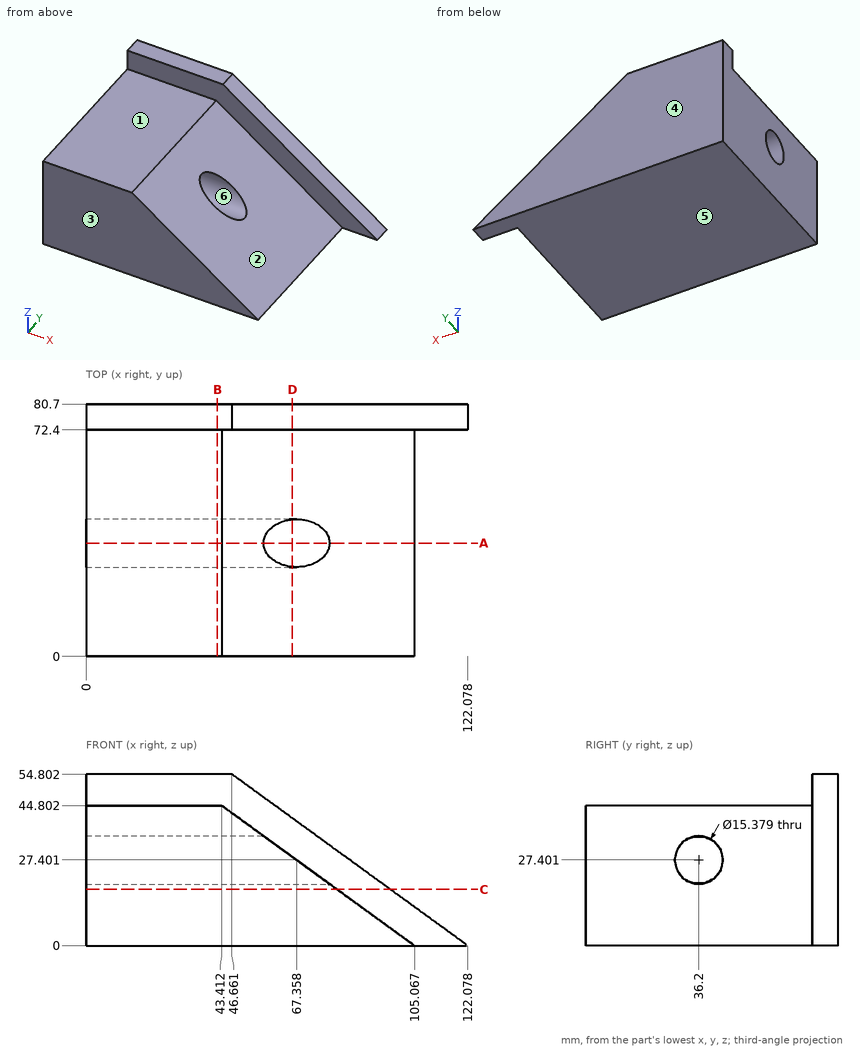
Input: dimensioned drawing with shaded views. Units: mm. Origin: part minimum x, y, z. A direction names the side the tool comes from. Round coordinates to 2 decimals unless told otherwise and drop trailing zeros. Order: outer loops, then holes, each group sorted by start corner. A loop starts at its lowest first (then second) coordinate and runs counter-clockwise, first axis right, second up. Notation, with made-up numbers: (6.25, 24.25) -> (15.25, 24.25) arc R16 cw to (15.25, 35.25) -> close; hole circle Ø7 at (-2, 69). An arc over 180 degrees is marked (long way). One line per item, written item: value. Start each with the question number.
Q1. Access query for the marked faces 1, 2 and 3. Directions: +Z, -Z, +X, -X, +Y, -Y. A direction counts if a zero-diameter tool reaches every point of the face in a straight line with its end or side. Return the directions, or none.
Q2. Section query D-D (x = 66). Return the cut outline in (y, z).
Q3. Draft query along Y for the marked faces 4, 5 and 6. Return one class per face: pulls with the +Y half, pulls with the -Y half, needs draft (parallel to the pull), parting line crosses it, or undercut.
Q4. Material intervals for probe 1 along Z at (x, y) = (42, 36.2); probe 2 along Z at (x, y) = (9, 66); probe 3 along Y at (x, z) = (55.5, 24) (1 decimal), sorted ascending.
Q5. Section query A-A (y = 36.2). Return the cut outline in (x, z), plus the area to 3 significant figures.
Q6. Section query B-B (x = 42). Return the cut outline in (y, z).
Q7. Pin query (flat end, axial travel): pin 1 (21.5 mm diameter, centred on x = 32, y = 45, fed in from +Z). Return the tip coordinate at first contact, or that it passes through.
Q8. Section query C-C (z = 18). Return the cut outline in (x, y) (1 decimal), plus the area to 3 significant figures.
Findings below:
1. face 1: +Z, +X, -X, -Y
1. face 2: +Z, +X, -Y
1. face 3: +Z, -Z, +X, -X, -Y
2. outline: (0, 0) -> (80.7, 0) -> (80.7, 40.75) -> (72.4, 40.75) -> (72.4, 28.39) -> (43.83, 28.39) arc R7.69 cw (long way) to (28.57, 28.39) -> (0, 28.39) -> close
3. face 4: pulls with the +Y half
3. face 5: needs draft
3. face 6: undercut
4. probe 1: 0 to 19.71, 35.09 to 44.8
4. probe 2: 0 to 44.8
4. probe 3: 0 to 29.3, 43.1 to 80.7
5. outline: (0, 0) -> (105.07, 0) -> (77.94, 19.71) -> (0, 19.71) -> close; (0, 35.09) -> (56.78, 35.09) -> (43.41, 44.8) -> (0, 44.8) -> close
5. area: 2,290 mm²
6. outline: (0, 0) -> (80.7, 0) -> (80.7, 54.8) -> (72.4, 54.8) -> (72.4, 44.8) -> (0, 44.8) -> close; hole circle Ø15.38 at (36.2, 27.4)
7. pin 1: z = 44.8
8. outline: (0, 0) -> (80.3, 0) -> (80.3, 72.4) -> (97.3, 72.4) -> (97.3, 80.7) -> (0, 80.7) -> close
8. area: 6,620 mm²
